For this review, take the finished solid that the model builds, in its own axes (mm). Face numbers are marked on the shaded views. A direction names the side the tool comes from. Round coordinates to 2 decimals unless told otherwise and drop trailing zeros. Loops run counter-clockwise (first coordinate to the right, second up) from the corner with the lowest first, then second, coordinate; pieces in that order, holes last.
1. Draft analysis for pull direction Y (two halves, no side actions). For the marked faces 4, 5 and 6, state which applies: released by +Y, released by -Y, zero draft, split by the parting line, or undercut.
2. Clearance check with flat-ended pins moving along their axes: pin 1 Ø8 at (x, z) = (6, 18.5) entering from -Y; pin 2 Ø12 at (y, z) = (-4, 20) entering from +X; pin 3 Ø3 at (x, y) = (-10.5, -7) entering from +Z. State where each tip first meets the part, or that it passes through.
3. Consider section A-A on z = 12.25. State the section outline as (x, y) points.
4. Tool access review of the marked faces 1, 2 and 3: name each direction out of +Z, -Z, +X, -X, +Y, -Y from which nothing blocks a thin tool from reaching the whole face with its end or side.
5. To check wall thickness, follow line 1 along Z through (x, y) = (-8, -2); line 2 along Z through (x, y) = (8, -2); line 3 along Y through (x, z) = (-1, 11). State the ranges of each line that lie inside material, in increasing order.
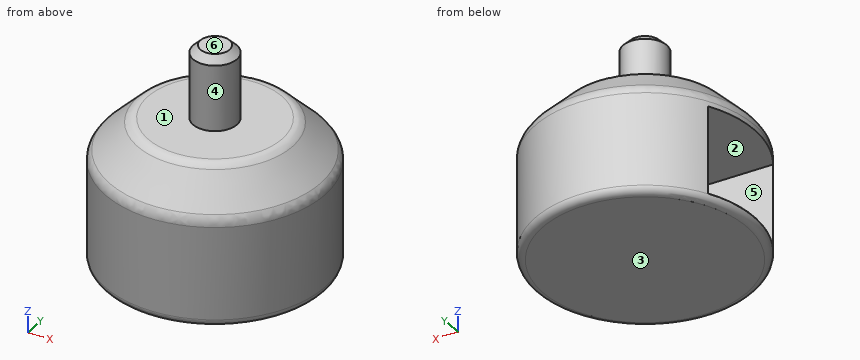
Autodesk Inventor part; units mm, degrees
ref_plane "Work Plane2" through (0, 14.5, 0) normal (0, 1, 0) x (-1, 0, 0)
ref_plane "Work Plane3" through (-14.75, 0, 0) normal (1, 0, 0) x (0, 1, 0)
ref_plane "XY Plane" through (0, 0, 0) normal (0, 0, 1) x (1, 0, 0)
sketch "Sketch1" plane through (0, 0, 0) normal (0, 0, 1) x (1, 0, 0)
  circle A0 centre (0, 0) radius 15
  dimension "d0" = 30
extrude "Extrusion1" add sketch "Sketch1" along normal blind 20
sketch "Sketch3" plane through (0, 0, 20) normal (0, 0, 1) x (1, 0, 0)
  circle A0 centre (0, 0) radius 15
extrude "Extrusion3" add sketch "Sketch3" along normal blind 1
chamfer "Chamfer1" distance 5 angle 45 1 edges at (-15, 0, 21)
fillet "Fillet1" radius 2 2 edges at (-15, 0, 16) (-10, 0, 21)
sketch "Sketch4" plane through (0, 0, 21) normal (0, 0, 1) x (1, 0, 0)
  circle A0 centre (0, 0) radius 3
  dimension "d12" = 6
extrude "Extrusion4" add sketch "Sketch4" along normal blind 10
chamfer "Chamfer2" distance 1 angle 45 1 edges at (-3, 0, 31)
fillet "Fillet2" radius 1 1 edges at (-15, 0, 0)
ref_plane "Work Plane2" through (0, 14.5, 0) normal (0, 1, 0) x (-1, 0, 0)
ref_plane "Work Plane1" through (0, -15.5, 0) normal (0, 1, 0) x (-1, 0, 0)
ref_plane "Work Plane3" through (-14.75, 0, 0) normal (1, 0, 0) x (0, 1, 0)
sketch "Sketch5" plane through (-14.75, 0, 0) normal (1, 0, 0) x (0, 1, 0)
  line L0 (7.5, 2.5) -> (-7.5, 2.5)
  line L1 (-7.5, 2.5) -> (-7.5, 14.5)
  line L2 (-7.5, 14.5) -> (7.5, 14.5)
  line L3 (7.5, 14.5) -> (7.5, 2.5)
  line L4 (9.8328, 18.3373) -> (9.8328, 18.1192)
  line L5 (7.5, 12.0972) -> (7.5, 12.3154)
  line L6 (-15, 1) -> (15, 1)
  line L7 (15, 1) -> (15, 15.1716)
  line L8 (-15, 1) -> (15, 1)
  line L9 (15, 1) -> (15, 15.1716)
  line L10 (15, 15.1716) -> (-15, 15.1716)
  line L11 (-15, 15.1716) -> (-15, 1)
  line L12 (15, 15.1716) -> (-15, 15.1716)
  point P0 (0, 0)
  dimension "d28" = 15
  dimension "d29" = 12
  dimension "d30" = 7.5
  dimension "d31" = 7.5
  dimension "d32" = 1.5
  dimension "d34" = 0
extrude "Extrusion5" cut sketch "Sketch5" along normal blind 20 and the other way blind 5 contours L0 L1 L2 L3
thread "Thread1"
sketch "Sketch6" plane through (5.25, 0, 0) normal (-1, 0, 0) x (0, 0, 1)
  line L0 (0, -16.1407) -> (1.4634, -16.1407)
  line L1 (1.4634, -16.1407) -> (1.4634, 17.2598)
  line L2 (1.4634, 17.2598) -> (0, 17.2598)
  line L3 (0, 17.2598) -> (0, -16.1407)
  point P0 (0, 0)
extrude "Extrusion6" cut sketch "Sketch6" along normal through all both and the other way through all
fillet "Fillet3" radius 1 1 edges at (-15, 0, 1.4634)
properties part number "Motor" material "UHMW, Black"
Resolved:
1. face 4: split by the parting line
1. face 5: undercut
1. face 6: zero draft
2. pin 1: stops at y = -14.6
2. pin 2: stops at x = 14.99
2. pin 3: stops at z = 19.88
3. outline: (-12.99, -7.5) arc R15 ccw (long way) to (-12.99, 7.5) - (5.25, 7.5) - (5.25, -7.5) - close
4. face 1: +Z
4. face 2: -X
4. face 3: -Z, +X, -X, +Y, -Y
5. line 1: z = 1.46 to 2.5, 14.5 to 21
5. line 2: z = 1.46 to 21
5. line 3: y = -14.97 to -7.5, 7.5 to 14.97
